from build123d import *

# Parameters (mm, degrees)
SKETCH_1_W          = 9
SKETCH_1_H          = 9
EXTRUDE_1_DEPTH     = 98
SKETCH_2_W          = 7
SKETCH_2_H          = 7
CUT_EXTRUDE_1_DEPTH = 106.6
SKETCH_3_R          = 1.5
CUT_EXTRUDE_2_DEPTH = 106.6
SKETCH_4_R          = 1.5
CUT_EXTRUDE_4_DEPTH = 50


with BuildPart() as part:
    # ｽｹｯﾁ1 → ﾎﾞｽ - 押し出し1 (new body)
    with BuildSketch(Plane.XY):
        Rectangle(SKETCH_1_W, SKETCH_1_H)
    extrude(amount=EXTRUDE_1_DEPTH)

    # ｽｹｯﾁ2 → ｶｯﾄ - 押し出し1 (cut)
    with BuildSketch(Plane.XY.offset(98)):
        Rectangle(SKETCH_2_W, SKETCH_2_H)
    extrude(amount=-CUT_EXTRUDE_1_DEPTH, mode=Mode.SUBTRACT)

    # ｽｹｯﾁ3 → ｶｯﾄ - 押し出し2 (cut)
    with BuildSketch(Plane(origin=(0, 4.5, 0), x_dir=(1, 0, 0), z_dir=(0, 1, 0))):
        with Locations((0, -93)):
            Circle(SKETCH_3_R)
        with Locations((0, -14)):
            Circle(SKETCH_3_R)
    extrude(amount=-CUT_EXTRUDE_2_DEPTH, mode=Mode.SUBTRACT)

    # ｽｹｯﾁ4 → ｶｯﾄ - 押し出し4 (cut)
    with BuildSketch(Plane.ZY.offset(4.5)):
        with Locations((5, 0)):
            Circle(SKETCH_4_R)
        with Locations((93, 0)):
            Circle(SKETCH_4_R)
    extrude(amount=-CUT_EXTRUDE_4_DEPTH, mode=Mode.SUBTRACT)


solid = part.part
CAD build for the part. Positions are in the model's coordinates, mm. A direction names the side the tool comes from. Coordinates: 2 decimals unless noted, no trailing zeros. Write each loop counter-clockwise with the first axis right and the second up, starting at its lowest first coordinate (ties: lowest second). Pieces come first, ordered by that corner, then holes. Notation, with made-up numbers: M 36,50.5 L 57,50.5 A30 ccw 57,81.5 Z; hole C -8.5,51 d5. An arc over 180 degrees is marked long. Answer as a JSON object with one key per item and string values. Group by question number.
1) Saw through at A-A (x = 0). Write the cut outline in (y, z).
2) Mould opens along Z. For faces 3 (the face through (-4.007, -0.575, 6.386)), 4 (the face through (-4, 0, 98)), 5 (the face through (-4, 0, 0)), 6 (the face through (-3.5, 0, 50)) say: +Z half, -Z half, draft (parallel to the pull), parting line (faces both ways), or undercut.
3) Pin check, flat tips, straight feed: pin 1 Ø4 at (x, z) = (0, 14) entering from -Y; pin 2 Ø1.8 at (y, z) = (0, 93) entering from +X. Stop position of each tip, or through.
4) Saw through at B-B (z = 42.5). Write the cut outline in (x, y).
5) Wall check: line 1 (Z direction, x = 0, y = 4.1); line 2 (X direction, y = 0, z = 47). Give the ranges that are in metal, low to high. Write a range as from..to.
6) Tool access for faces 1 (the face through (-4.01, 0.45, 94.43)), 2 (the face through (0, -3.5, 50)): list every direction of +Z, -Z, +X, -X, +Y, -Y with a clear straight run to the whole face (end or side of a thin tool).
7) Saw through at D-D (y = 0). Write the cut outline in (x, z), plus the area to 3 significant figures.
8) Saw through at C-C (z = 93). Write the cut outline in (x, y).
Values follow:
{
 "1": {"outline": "M -4.5,0 L -3.5,0 L -3.5,12.5 L -4.5,12.5 Z; M -4.5,15.5 L -3.5,15.5 L -3.5,91.5 L -4.5,91.5 Z; M -4.5,94.5 L -3.5,94.5 L -3.5,98 L -4.5,98 Z; M 3.5,0 L 4.5,0 L 4.5,12.5 L 3.5,12.5 Z; M 3.5,15.5 L 4.5,15.5 L 4.5,91.5 L 3.5,91.5 Z; M 3.5,94.5 L 4.5,94.5 L 4.5,98 L 3.5,98 Z"},
 "2": {"face 3": "undercut", "face 4": "+Z half", "face 5": "-Z half", "face 6": "draft"},
 "3": {"pin 1": "stops at y = -4.5", "pin 2": "passes through"},
 "4": {"outline": "M -4.5,-4.5 L 4.5,-4.5 L 4.5,4.5 L -4.5,4.5 Z; hole M -3.5,-3.5 L 3.5,-3.5 L 3.5,3.5 L -3.5,3.5 Z"},
 "5": {"line 1": "z = 0..12.5, 15.5..91.5, 94.5..98", "line 2": "x = -4.5..-3.5, 3.5..4.5"},
 "6": {"face 1": "+X, -X", "face 2": "+Z, -Z"},
 "7": {"outline": "M -4.5,0 L -3.5,0 L -3.5,3.5 L -4.5,3.5 Z; M -4.5,6.5 L -3.5,6.5 L -3.5,91.5 L -4.5,91.5 Z; M -4.5,94.5 L -3.5,94.5 L -3.5,98 L -4.5,98 Z; M 3.5,0 L 4.5,0 L 4.5,3.5 L 3.5,3.5 Z; M 3.5,6.5 L 4.5,6.5 L 4.5,91.5 L 3.5,91.5 Z; M 3.5,94.5 L 4.5,94.5 L 4.5,98 L 3.5,98 Z", "area": "184 mm2"},
 "8": {"outline": "M -4.5,-4.5 L -1.5,-4.5 L -1.5,-3.5 L -3.5,-3.5 L -3.5,-1.5 L -4.5,-1.5 Z; M -4.5,1.5 L -3.5,1.5 L -3.5,3.5 L -1.5,3.5 L -1.5,4.5 L -4.5,4.5 Z; M 1.5,-4.5 L 4.5,-4.5 L 4.5,-1.5 L 3.5,-1.5 L 3.5,-3.5 L 1.5,-3.5 Z; M 1.5,3.5 L 3.5,3.5 L 3.5,1.5 L 4.5,1.5 L 4.5,4.5 L 1.5,4.5 Z"}
}
